Verification items for this drawing (mm, ordinates from the low corner). Round coordinates to 2 decimals unless told otherwise and drop trailing zeros. Loops run counter-clockwise (first coordinate to the right, second up) from the corner with the lowest first, then second, coordinate; pieces in that order, holes last. Notation, with made-up numbers: M -4.75,47 L 26.25,47 A16 cw 26.25,55 Z; hole C -7.75,54 d9. An arc over 180 degrees is marked long. Answer in a Markdown table with one row per item. Add a question column.
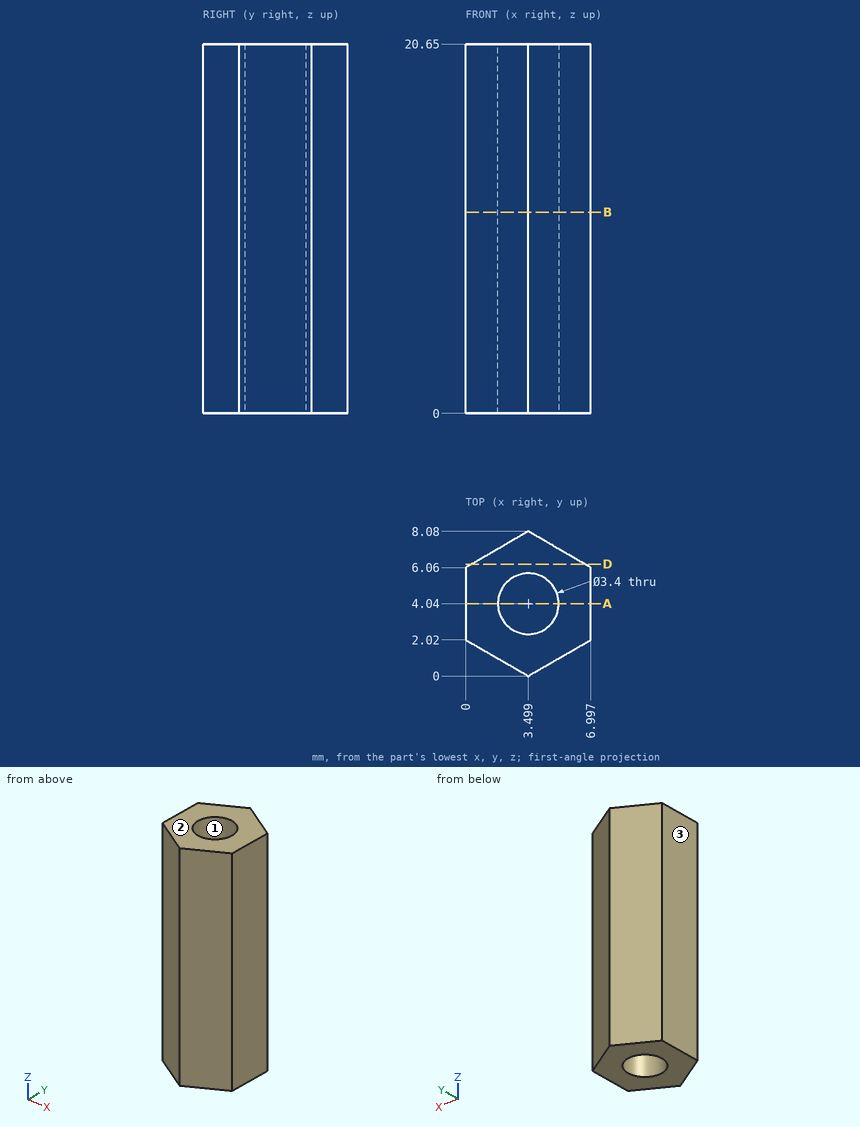
1) Cross-section at B-B, the plane z = 11.25. Record the boundary of the cut face in (x, y).
2) Draft check along X on the marked faces 1, 2 and 3. Enter one of: +X half, -X half, draft (parallel to the pull), parting line (faces both ways), or undercut.
3) Cross-section at D-D, the plane y = 6.25. Record the boundary of the cut face in (x, z).
4) Go/stop test with a flat-tipped pin: pin 1 (1 mm diameter, centred on x = 2.5, z = 7, fed in from -Y). Record where the tip stops, or that it passes through.
5) Thickness scan on L1, parallel to X at y = 4.04, z = 16; L2, parallel to Y at x = 3.25, z = 6 (1 decimal); L3, parallel to X at y = 3.25, z = 8 (1 decimal). Record the ranges inside material, lowest first. Write a range as [from, to].
6) Cross-section at A-A, the plane y = 4.04. Record the boundary of the cut face in (x, z).
Worked answers:
| question | item | result |
|---|---|---|
| 1 | outline | M 0,2.02 L 3.5,0 L 7,2.02 L 7,6.06 L 3.5,8.08 L 0,6.06 Z; hole C 3.5,4.04 d3.4 |
| 2 | face 1 | undercut |
| 2 | face 2 | draft |
| 2 | face 3 | -X half |
| 3 | outline | M 0.33,0 L 6.67,0 L 6.67,20.65 L 0.33,20.65 Z |
| 4 | pin 1 | stops at y = 0.29 |
| 5 | L1 | x = [0, 1.8], [5.2, 7] |
| 5 | L2 | y = [0.1, 2.4], [5.7, 7.9] |
| 5 | L3 | x = [0, 2], [5, 7] |
| 6 | outline | M 0,0 L 1.8,0 L 1.8,20.65 L 0,20.65 Z; M 5.2,0 L 7,0 L 7,20.65 L 5.2,20.65 Z |
